Here's the drawing with two shaded views (mm, measured from the low corner). I have some questions. Give positions to 0.01 mm unless a question says otherwise; leave off trailing zeros. Loops run counter-clockwise (first coordinate to the right, second up) from the corner with the lowest first, then second, coordinate; pieces in that order, holes last.
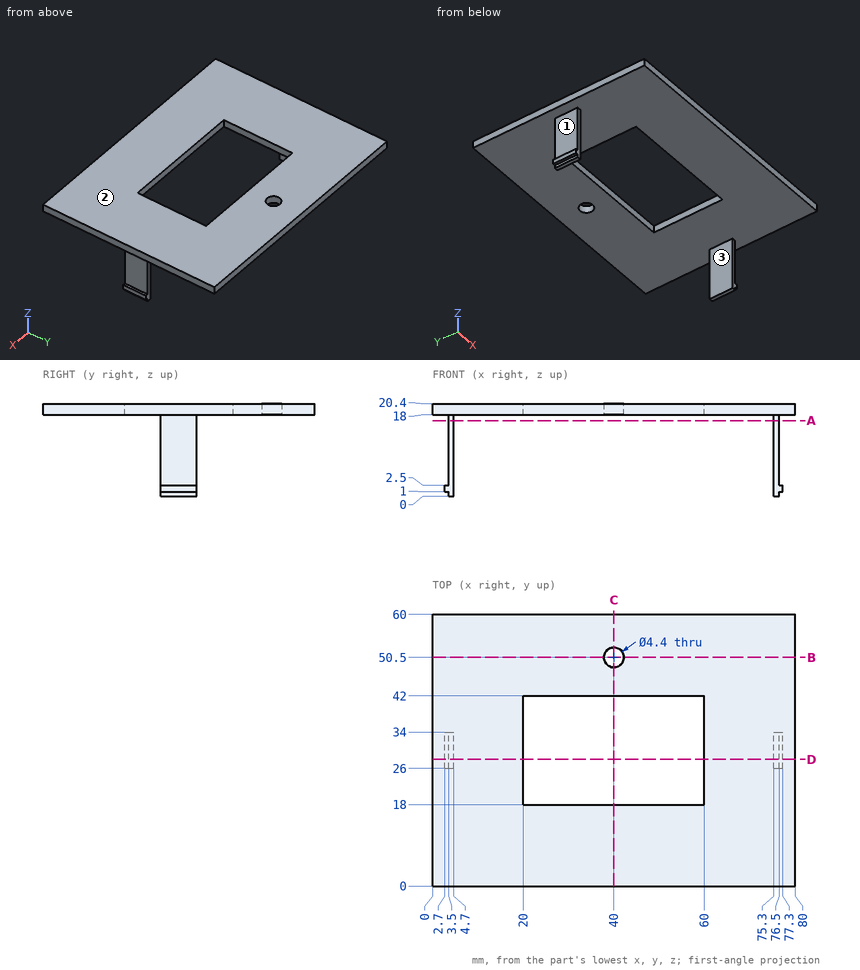
(1) Please list where these lines run through material, in increasing order: probe 1 along X at (y, z) = (50.5, 19.7); probe 2 along Y at (x, z) = (40, 19.6); probe 3 along X at (y, z) = (27.5, 12.75).
Returned:
probe 1: x = 0 to 37.8, 42.2 to 80
probe 2: y = 0 to 18, 42 to 48.3, 52.7 to 60
probe 3: x = 3.5 to 4.7, 75.3 to 76.5
(2) Suppose I cut it at A-A on z = 16.75. List the corners of the cut face in (x, y) for me, plus the area to 3 significant figures.
Returned:
outline: (3.5, 26) - (4.7, 26) - (4.7, 34) - (3.5, 34) - close; (75.3, 26) - (76.5, 26) - (76.5, 34) - (75.3, 34) - close
area: 19.2 mm2
(3) Will these pins go through, and if not, where does the flat tip stop? P1, Ø2.5, axis at y = 29.5, z = 13.5, coming from the +X side; P2, Ø5.5, axis at x = 40, y = 50.5, coming from the +Z side; P3, Ø2, axis at x = 76, z = 12.5, coming from the -Y side; P4, Ø0.9, axis at x = 3, y = 31, coming from the -Z side.
Returned:
P1: stops at x = 76.5
P2: stops at z = 20.4
P3: stops at y = 26
P4: stops at z = 1
(4) Suppose I cut it at B-B on y = 50.5. List the corners of the cut face in (x, z) for me.
Returned:
outline: (0, 18) - (37.8, 18) - (37.8, 20.4) - (0, 20.4) - close; (42.2, 18) - (80, 18) - (80, 20.4) - (42.2, 20.4) - close
(5) Thinking about a two-plate mould opening in Z: for the marked faces 1, 2 and 3, which applies, pulls with the +Z half, pulls with the -Z half, needs draft (parallel to the pull), parting line crosses it, or undercut?
Returned:
face 1: undercut
face 2: pulls with the +Z half
face 3: needs draft
(6) Suppose I cut it at C-C on x = 40. List the corners of the cut face in (y, z) for me, plus the area to 3 significant figures.
Returned:
outline: (0, 18) - (18, 18) - (18, 20.4) - (0, 20.4) - close; (42, 18) - (48.3, 18) - (48.3, 20.4) - (42, 20.4) - close; (52.7, 18) - (60, 18) - (60, 20.4) - (52.7, 20.4) - close
area: 75.8 mm2
(7) Suppose I cut it at D-D on y = 28. List the corners of the cut face in (x, z) for me, plus the area to 3 significant figures.
Returned:
outline: (0, 18) - (3.5, 18) - (3.5, 2.5) - (2.7, 2.5) - (2.7, 1) - (3.5, 1) - (3.5, 0) - (4.7, 0) - (4.7, 18) - (20, 18) - (20, 20.4) - (0, 20.4) - close; (60, 18) - (75.3, 18) - (75.3, 0) - (76.5, 0) - (76.5, 1) - (77.3, 1) - (77.3, 2.5) - (76.5, 2.5) - (76.5, 18) - (80, 18) - (80, 20.4) - (60, 20.4) - close
area: 142 mm2
